Design review of the part built by this model. Coordinates are the model's own, in mm. A direction names the side the tool comes from. Give positions to 0.01 mm unless a question says otherwise; leave off trailing zeros. Write each loop counter-clockwise with the first axis right and the second up, starting at its lowest first coordinate (ties: lowest second). Pieces come first, ordered by that corner, then holes. Notation, with made-up numbers: (28, 49.5) -> (41, 49.5) arc R16 ccw to (41, 69.5) -> close; hole circle Ø2 at (47.25, 81.25). An arc over 180 degrees is marked (long way). Put each result on its own line as item: value. Start each with the question number.
from build123d import *

# Parameters (mm, degrees)
SKETCH_1_W           = 20.18
SKETCH_1_H           = 9
EXTRUDE_1_DEPTH      = 9
SKETCH_2_W           = 17.78
SKETCH_2_H           = 6.6
CUT_EXTRUDE_1_DEPTH  = 6.5
SKETCH_3_W           = 4.2
SKETCH_3_H           = 6.5
CUT_EXTRUDE_2_DEPTH  = 6.5
EXTRUDE_2_DEPTH      = 3.5
EXTRUDE_2_DEPTH_BACK = 8
SKETCH_5_W           = 0.75
SKETCH_5_H           = 0.75


with BuildPart() as part:
    # 草图1 → 拉伸1 (new body)
    with BuildSketch(Plane(origin=(0, 0, 0), x_dir=(1, 0, 0), z_dir=(0, 1, 0))):
        Rectangle(SKETCH_1_W, SKETCH_1_H)
    extrude(amount=EXTRUDE_1_DEPTH)

    # 草图2 → 切除-拉伸1 (cut)
    with BuildSketch(Plane(origin=(0, 9, 0), x_dir=(-1, 0, 0), z_dir=(0, 1, 0))):
        Rectangle(SKETCH_2_W, SKETCH_2_H)
    extrude(amount=-CUT_EXTRUDE_1_DEPTH, mode=Mode.SUBTRACT)

    # 草图3 → 切除-拉伸2 (cut)
    with BuildSketch(Plane.XY.offset(4.5)):
        with Locations((0, 5.75)):
            Rectangle(SKETCH_3_W, SKETCH_3_H)
    extrude(amount=-CUT_EXTRUDE_2_DEPTH, mode=Mode.SUBTRACT)

    # 草图5 → 拉伸2 (add, two sides: drawn at the far end of the back side and taken through both)
    with BuildSketch(Plane.XZ.offset(-EXTRUDE_2_DEPTH_BACK)):
        with Locations((0, 1.27)):
            Rectangle(SKETCH_5_W, SKETCH_5_H)
        with Locations((2.54, 1.27)):
            Rectangle(SKETCH_5_W, SKETCH_5_H)
        with Locations((5.08, 1.27)):
            Rectangle(SKETCH_5_W, SKETCH_5_H)
        with Locations((-2.54, 1.27)):
            Rectangle(SKETCH_5_W, SKETCH_5_H)
        with Locations((-5.08, 1.27)):
            Rectangle(SKETCH_5_W, SKETCH_5_H)
        with Locations((-5.08, -1.27)):
            Rectangle(SKETCH_5_W, SKETCH_5_H)
        with Locations((-2.54, -1.27)):
            Rectangle(SKETCH_5_W, SKETCH_5_H)
        with Locations((5.08, -1.27)):
            Rectangle(SKETCH_5_W, SKETCH_5_H)
        with Locations((2.54, -1.27)):
            Rectangle(SKETCH_5_W, SKETCH_5_H)
        with Locations((0, -1.27)):
            Rectangle(SKETCH_5_W, SKETCH_5_H)
    extrude(amount=EXTRUDE_2_DEPTH + EXTRUDE_2_DEPTH_BACK)


solid = part.part
Q1. To check wall thickness, follow probe 1 along Z at (x, y) = (-5, 3.5) (3 decimals); probe 2 along Z at (x, y) = (8.5, 4); probe 3 along X at (y, z) = (4.5, -0.5). State the ranges of each line that lie inside material, in increasing order. Write a range as from..to.
Q2. Take a section at C-C on z = -0.25. Give the boundary of the cut face in (x, y), then the cut area to 4 significant figures.
Q3. Take a section at B-B on y = 6.75. State how many separate pieces and enclosed holes the cut face has, then the cut area to 3 significant figures.
Q4. Machinability: for faces 1 (the face through (0, 2, 4.5)), 2 (the face through (2.1, 6, 4)), 3 (the face through (-5, 6, 3.3)), which of the approach directions +Z, -Z, +X, -X, +Y, -Y give a long, thin tool a straight path to every point of the face, cutting with its end or side? Answer none if there is none.
Q5. For pin 1 (0.8 mm diameter, centred on x = 0, z = -1, fed in from +Y); pin 2 (0.6 mm diameter, centred on y = -2, z = -1.5, fed in from +X) (3 decimals); pin 3 (0.6 mm diameter, centred on x = -5, y = -2.5, fed in from -Z) (3 decimals), all flat-tipped, find the tip position at first contact; note any pin that passes through.
Q6. Take a section at A-A on x = 3.25. Give the boundary of the cut face in (y, z).
Q7. Mouldability with a two-part tool opening along X and no side actions: class faces 4 (the face through (-0.1, 2.5, 0.7)), 5 (the face through (10.09, 4, 0)), 6 (the face through (-2, 9, -4)) as +X half, -X half, draft (parallel to the pull), parting line (faces both ways), or undercut.
Result:
1. probe 1: z = -4.5..-3.3, -1.645..-0.895, 0.895..1.645, 3.3..4.5
1. probe 2: z = -4.5..-3.3, 3.3..4.5
1. probe 3: x = -10.09..-8.89, 8.89..10.09
2. outline: (-10.09, 0) -> (10.09, 0) -> (10.09, 9) -> (8.89, 9) -> (8.89, 2.5) -> (-8.89, 2.5) -> (-8.89, 9) -> (-10.09, 9) -> close
2. area: 66.05 mm^2
3. separate pieces: 11
3. enclosed holes: 0
3. area: 64.9 mm^2
4. face 1: +Z, +X, -X, +Y, -Y
4. face 2: +Z, +Y
4. face 3: +Y
5. pin 1: stops at y = 8
5. pin 2: stops at x = 5.455
5. pin 3: stops at z = -1.645
6. outline: (0, -4.5) -> (9, -4.5) -> (9, -3.3) -> (2.5, -3.3) -> (2.5, 3.3) -> (9, 3.3) -> (9, 4.5) -> (0, 4.5) -> close
7. face 4: undercut
7. face 5: +X half
7. face 6: draft
